from build123d import *

# Parameters (mm, degrees)
F0_W        = 3.4
F0_H        = 3.4
F1_DEPTH    = 27
F2_SIZE     = 1
F3_W        = 4.9
F3_H        = 2
F4_DEPTH    = 10
F5_T4_DEPTH = 22.5734639037
F7_DEPTH    = 5


# Not quite as in the source:
# - a fillet or chamfer that OpenCascade refuses, or shapes differently, is made with other operations: its cross-section is extruded or revolved along the edge and cut away or added


with BuildPart() as f1:
    # F0 (on Top) → F1 (new body)
    with BuildSketch(Plane.XY):
        Rectangle(F0_W, F0_H)
    extrude(amount=F1_DEPTH)

    # F2
    f2_edges = [f1.edges().sort_by_distance(p)[0] for p in [
        (-1.7, 0, 27),
    ]]
    chamfer(f2_edges, length=F2_SIZE)

    # F3 (on face) → F4 (join)
    with BuildSketch(Plane.YZ.offset(1.7)):
        with Locations((-0.75, 26)):
            Rectangle(F3_W, F3_H)
    extrude(amount=F4_DEPTH)

    # F5: chamfer of 4 on 1 edges, made by hand


with BuildPart() as f5_tool2:
    # F5_s3 → F5_t4 (new body)
    with BuildSketch(Plane.XY.offset(37.2867319519)):
        Polygon((1.7, 0.8), (5.7, -3.2), (1.7, -3.2), align=None)
    extrude(amount=-F5_T4_DEPTH)

    split(bisect_by=Plane.XZ.offset(1.7), keep=Keep.TOP)


with BuildPart() as f1_1:
    add(f1.part)

    # F5_t1: cut F5_tool2
    add(f5_tool2.part, mode=Mode.SUBTRACT)

    # F6 (on face) → F7 (join)
    with BuildSketch(Plane.XY):
        with BuildLine():
            ThreePointArc((0, -1.7), (1.202081528, -1.202081528), (1.7, 0))
            ThreePointArc((1.7, 0), (1.202081528, 1.202081528), (0, 1.7))
            ThreePointArc((0, 1.7), (-1.202081528, 1.202081528), (-1.7, 0))
            ThreePointArc((-1.7, 0), (-1.202081528, -1.202081528), (0, -1.7))
        make_face()
    extrude(amount=-F7_DEPTH)

    # F8: chamfer of 0.4 on 1 edges, made by hand

    # F8_s1 → F8_t2 (revolve, cut)
    with BuildSketch(Plane.XZ):
        Polygon((-1.7, -4.6), (-1.3, -5), (-1.7, -5), align=None)
    revolve(axis=Axis((0, 0, -5), (0, 0, 1)), mode=Mode.SUBTRACT)


solid = f1_1.part
Part model, mm, in its own coordinate system. A direction names the side the tool comes from. Give positions to 0.01 mm unless a question says otherwise; leave off trailing zeros. Loops run counter-clockwise (first coordinate to the right, second up) from the corner with the lowest first, then second, coordinate; pieces in that order, holes last. Notation, with made-up numbers: M 68,-16 L 100,-16 A3 ccw 100,-12 Z; hole C -20.75,8 d2. An arc over 180 degrees is marked long. Put each result on its own line as item: value. Start each with the question number.
1) Saw through at B-B (x = 8). List the corners of the cut face in (y, z).
2) 3-axis set-ups, long thin cutter, end or side, ignore diameter. For faces 1 (the flat face through (1.7, 0, 12)), 2 (the flat face through (-1.4, -1.3, 0)), 3 (the flat face through (1.3, 1.4, 0)), 4 (the flat face through (1.35, -1.35, 0)): which of +Z, -Z, +X, -X, +Y, -Y reach the whole face in a straight line?
3) Flat gauge pins, fed straight in: pin 1 (4.5 mm diameter, centred on x = 1, z = 16, fed in from -Y); pin 2 (2.5 mm diameter, centred on y = 0.5, z = 11.5, fed in from +X); pin 3 (2.5 mm diameter, centred on x = 6.5, y = -0.5, fed in from -Z); pin 4 (8 mm diameter, centred on x = 9.5, z = -1, fed in from -Y). Where does each tip first touch, or does it go through?
4) Probe probe 1 along Z at (x, y) = (2, -1.6); probe 2 along X at (y, z) = (0.3, 20.5). List the from-to ranges inside material, lowest first.
5) Saw through at A-A (z = 24). List the corners of the cut face in (x, y).
6) Saw through at C-C (z = -1.5). List the corners of the cut face in (x, y).
Numbers:
1. outline: M -3.2,25 L 1.7,25 L 1.7,27 L -3.2,27 Z
2. face 1: -Z, +X, +Y, -Y
2. face 2: -Z, -X, -Y
2. face 3: -Z, +X, +Y
2. face 4: -Z, +X, -Y
3. pin 1: y = -1.7
3. pin 2: x = 1.7
3. pin 3: z = 25
3. pin 4: through
4. probe 1: 25 to 27
4. probe 2: -1.7 to 1.7
5. outline: M -1.7,-1.7 L 1.7,-1.7 L 1.7,1.7 L -1.7,1.7 Z
6. outline: C 0,0 d3.4
